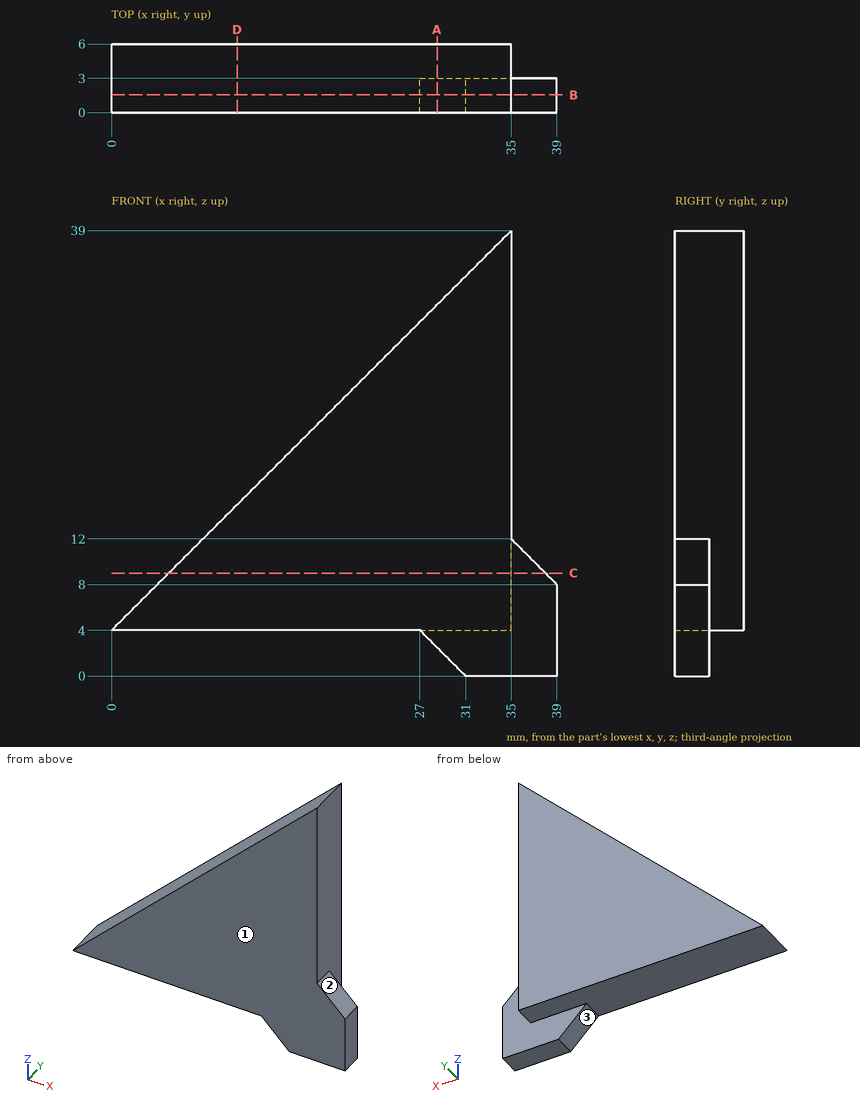
Source: three-view drawing plus pictorial views. Frame: mm from the lowest corner of the part. Round coordinates to 2 decimals unless told otherwise and drop trailing zeros. Loops run counter-clockwise (first coordinate to the right, second up) from the corner with the lowest first, then second, coordinate; pieces in that order, holes last. Notation, with made-up numbers: (-29, -26.75) - (3, -26.75) arc R20 ccw to (3, -4.75) - close; hole circle Ø9 at (32, 31.5). An arc over 180 degrees is marked (long way). Write item = value, one per line. Start each with the question number.
Item 1: Section query A-A on x = 28.5. Output: boundary loops of the cut face in (y, z), plus the area to 4 significant figures.
Item 2: Section query B-B on y = 1.55. Output: boundary loops of the cut face in (x, z), plus the area to 4 significant figures.
Item 3: Section query D-D on x = 11. Output: boundary loops of the cut face in (y, z).
Item 4: Mould query, pull axis X, two halves, no side actions, for the marked faces 1, 2 and 3. Classes: released by +X, released by -X, zero draft, split by the parting line, or undercut.
Item 5: Section query C-C on z = 9. Output: boundary loops of the cut face in (x, y).
Item 6: First-contact query: pin 1 Ø1.5 at (x, z) = (12.5, 19) entering from +Y; pin 2 Ø2 at (x, y) = (23.5, 4.5) entering from +Z; pin 3 Ø1.5 at (y, z) = (2.5, 34.5) entering from +X; pin 4 Ø2 at (x, y) = (14, 1.5) entering from +Z. Flat tips, straight axial feed; report the tip coordinate or a pass-through.
Item 7: Material intervals for line 1 (Z direction, x = 4, y = 2.95); line 2 (Y direction, x = 31.5, z = 3.5); line 3 (X direction, y = 5.6, z = 13), sorted ascending.
Results list:
q1.outline = (0, 2.5) - (3, 2.5) - (3, 4) - (6, 4) - (6, 32.5) - (0, 32.5) - close
q1.area = 175.5 mm²
q2.outline = (0, 4) - (27, 4) - (31, 0) - (39, 0) - (39, 8) - (35, 12) - (35, 39) - close
q2.area = 676.5 mm²
q3.outline = (0, 4) - (6, 4) - (6, 15) - (0, 15) - close
q4.face_1 = zero draft
q4.face_2 = released by +X
q4.face_3 = released by -X
q5.outline = (5, 0) - (38, 0) - (38, 3) - (35, 3) - (35, 6) - (5, 6) - close
q6.pin_1 = through
q6.pin_2 = 28.5
q6.pin_3 = 35
q6.pin_4 = 19
q7.line_1 = 4 to 8
q7.line_2 = 0 to 3
q7.line_3 = 9 to 35
